```python
from build123d import *

# Parameters (mm, degrees)
ESQUISSE1_R        = 50
ESQUISSE1_R_2      = 3.6
ESQUISSE1_R_3      = 2.05
ESQUISSE1_R_4      = 1.55
BOSS_EXTRU_1_DEPTH = 5
SKETCH4_R          = 38
CUT_EXTRUDE3_DEPTH = 10


with BuildPart() as part:
    # Esquisse1 → Boss.-Extru.1 (new body)
    with BuildSketch(Plane.XY):
        Circle(ESQUISSE1_R)
        with Locations((-40.096976195, -23.15)):
            Circle(ESQUISSE1_R_2, mode=Mode.SUBTRACT)
        with Locations((-40.096976195, 23.15)):
            Circle(ESQUISSE1_R_2, mode=Mode.SUBTRACT)
        with Locations((0, 46.3)):
            Circle(ESQUISSE1_R_2, mode=Mode.SUBTRACT)
        with Locations((40.096976195, 23.15)):
            Circle(ESQUISSE1_R_2, mode=Mode.SUBTRACT)
        with Locations((40.096976195, -23.15)):
            Circle(ESQUISSE1_R_2, mode=Mode.SUBTRACT)
        with Locations((0, -46.3)):
            Circle(ESQUISSE1_R_2, mode=Mode.SUBTRACT)
        with Locations((0, 19.165334425)):
            Circle(ESQUISSE1_R_3, mode=Mode.SUBTRACT)
        with Locations((0, -19.232757636)):
            Circle(ESQUISSE1_R_3, mode=Mode.SUBTRACT)
        with Locations((-33.234018716, 33.234018716)):
            Circle(ESQUISSE1_R_4, mode=Mode.SUBTRACT)
        with Locations((33.234018716, 33.234018716)):
            Circle(ESQUISSE1_R_4, mode=Mode.SUBTRACT)
        with Locations((33.234018716, -33.234018716)):
            Circle(ESQUISSE1_R_4, mode=Mode.SUBTRACT)
        with Locations((-33.234018716, -33.234018716)):
            Circle(ESQUISSE1_R_4, mode=Mode.SUBTRACT)
        with Locations((-16.671397033, -9.625235564)):
            Circle(ESQUISSE1_R_3, mode=Mode.SUBTRACT)
        with Locations((16.669571796, 9.624181764)):
            Circle(ESQUISSE1_R_3, mode=Mode.SUBTRACT)
        with Locations((-16.671397032, 9.625235564)):
            Circle(ESQUISSE1_R_3, mode=Mode.SUBTRACT)
        with Locations((16.666666667, -9.622504487)):
            Circle(ESQUISSE1_R_3, mode=Mode.SUBTRACT)
    extrude(amount=BOSS_EXTRU_1_DEPTH)

    # Sketch4 → Cut-Extrude3 (cut)
    with BuildSketch(Plane(origin=(0, 0, 0), x_dir=(-1, 0, 0), z_dir=(0, 0, -1))):
        Circle(SKETCH4_R)
    extrude(amount=-CUT_EXTRUDE3_DEPTH, mode=Mode.SUBTRACT)


solid = part.part
```
The listing builds one solid part. Answer for the finished solid, in the listing's coordinates (mm). Round coordinates to 2 decimals unless told otherwise and drop trailing zeros. Loops run counter-clockwise (first coordinate to the right, second up) from the corner with the lowest first, then second, coordinate; pieces in that order, holes last.
Q1. Find the intervals of material crossed by line 1 (Y direction, x = 42, z = 1.85); line 2 (Y direction, x = 38.5, z = 2); line 3 (Y direction, x = -34.5, z = 3.6), in increasing order.
Q2. For a pull along X with two mould halves and no side action, classify faces 1 (the face through (-19, 34, 5)), 2 (the face through (47.69, 15.02, 2.46)), 3 (the face through (31.686, 33.302, 2.465)), 4 (the face through (-32.401, -31.927, 2.465)) as released by +X, released by -X, zero draft, split by the parting line, or undercut.
Q3. Given pin 1 Ø2 at (x, z) = (33, 1) entering from -Y; pin 2 Ø3 at (x, y) = (-33.23, 33.23) entering from -Z; pin 3 Ø3 at (x, z) = (4.5, 2.5) entering from +Y; pin 4 Ø1.5 at (y, z) = (3.5, 2.5) entering from +X, each flat-ended and moving along its own axis, determine where each tip first touches the part or whether it passes through.
Q4. Section C-C, the plane x = -20 is taken. Determine the outline of the cut face in (y, z).
Q5. Section D-D, the plane z = 3.7 is taken. Count the separate pieces of the cut face and the enclosed holes in it, then the cut area to 3 significant figures.
Q6. Section A-A, the plane y = 0 is taken. Determine the outline of the cut face in (x, z), then the cut area to 3 significant figures.
Q7. Section B-B, the plane x = 0 is taken. Determine the outline of the cut face in (y, z).
Completed:
1. line 1: y = -27.13 to -26.21, -20.09 to 20.09, 26.21 to 27.13
1. line 2: y = -31.9 to -26.38, -19.92 to 19.92, 26.38 to 31.9
1. line 3: y = -36.19 to -34.13, -32.34 to -15.93, 15.93 to 32.34, 34.13 to 36.19
2. face 1: zero draft
2. face 2: split by the parting line
2. face 3: undercut
2. face 4: undercut
3. pin 1: stops at y = -38.42
3. pin 2: passes through
3. pin 3: stops at y = 49.91
3. pin 4: stops at x = 49.92
4. outline: (-45.83, 0) - (-32.31, 0) - (-32.31, 5) - (-45.83, 5) - close; (32.31, 0) - (45.83, 0) - (45.83, 5) - (32.31, 5) - close
5. separate pieces: 1
5. enclosed holes: 11
5. area: 3,040 mm2
6. outline: (-50, 0) - (-38, 0) - (-38, 5) - (-50, 5) - close; (38, 0) - (50, 0) - (50, 5) - (38, 5) - close
6. area: 120 mm2
7. outline: (-50, 0) - (-49.9, 0) - (-49.9, 5) - (-50, 5) - close; (-42.7, 0) - (-38, 0) - (-38, 5) - (-42.7, 5) - close; (38, 0) - (42.7, 0) - (42.7, 5) - (38, 5) - close; (49.9, 0) - (50, 0) - (50, 5) - (49.9, 5) - close
